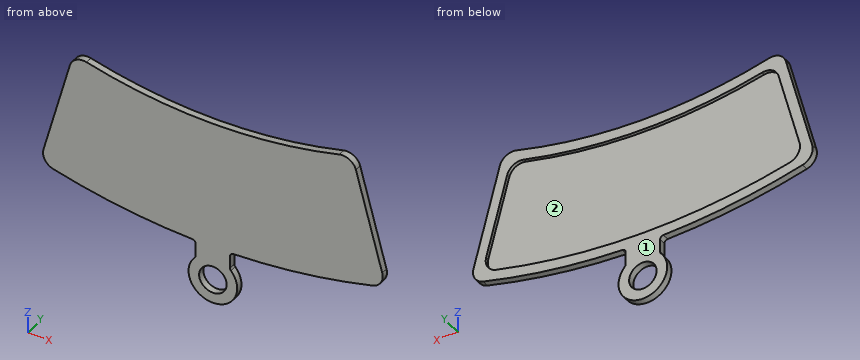
from build123d import *

# Parameters (mm, degrees)
BOSS_EXTRUDE1_DEPTH   = 1
CUT_EXTRUDE2_DEPTH    = 0.5
FILLET2_R             = 2
FILLET3_R             = 0.5
F_4_0MM_DOWEL_HOLE1_D = 4


with BuildPart() as part:
    # Sketch1 → Boss-Extrude1 (new body)
    with BuildSketch(Plane(origin=(0, 0, 0), x_dir=(1, 0, 0), z_dir=(0, 1, 0))):
        with BuildLine():
            Line((-25.127648951, 87.982107603), (-20.261027783, 69.819630142))
            ThreePointArc((-20.261027783, 69.819630142), (0, 72.7), (20.261027783, 69.819630142))
            Line((20.261027783, 69.819630142), (25.127648951, 87.982107603))
            ThreePointArc((25.127648951, 87.982107603), (13.92309714, 90.434492126), (2.499766704, 91.465846995))
            Line((2.499766704, 91.465846995), (2.499766704, 94))
            ThreePointArc((2.499766704, 94), (0.000164965, 100.03536894), (-2.5, 94.000233296))
            Line((-2.5, 94.000233296), (-2.5, 91.465840618))
            ThreePointArc((-2.5, 91.465840618), (-13.923212473, 90.434474369), (-25.127648951, 87.982107603))
        make_face()
    extrude(amount=BOSS_EXTRUDE1_DEPTH)

    # Sketch2 → Cut-Extrude2 (cut)
    with BuildSketch(Plane(origin=(0, 1, 0), x_dir=(1, 0, 0), z_dir=(0, 1, 0))):
        with BuildLine():
            Line((19.204373147, 71.671696311), (23.293714059, 86.933324366))
            ThreePointArc((23.293714059, 86.933324366), (0, 90), (-23.293714059, 86.933324366))
            Line((-23.293714059, 86.933324366), (-19.204373147, 71.671696311))
            ThreePointArc((-19.204373147, 71.671696311), (0, 74.2), (19.204373147, 71.671696311))
        make_face()
    extrude(amount=-CUT_EXTRUDE2_DEPTH, mode=Mode.SUBTRACT)

    # Fillet2
    fillet2_edges = [part.edges().sort_by_distance(p)[0] for p in [
        (25.127648951, 0.5, -87.982107603),
        (20.261027783, 0.5, -69.819630142),
        (-20.261027783, 0.5, -69.819630142),
        (-25.127648951, 0.5, -87.982107603),
        (19.204373147, 0.75, -71.671696311),
        (-19.204373147, 0.75, -71.671696311),
        (-23.293714059, 0.75, -86.933324366),
        (23.293714059, 0.75, -86.933324366),
    ]]
    fillet(fillet2_edges, radius=FILLET2_R)

    # Fillet3
    fillet3_edges = [part.edges().sort_by_distance(p)[0] for p in [
        (-2.5, 0.5, -91.465840618),
        (-2.5, 0.5, -94.000233296),
        (2.499766704, 0.5, -94),
        (2.499766704, 0.5, -91.465846995),
    ]]
    fillet(fillet3_edges, radius=FILLET3_R)

    # Ø4.0mm Dowel Hole1 (through all)
    with Locations(Plane(origin=(0, 1, 0), x_dir=(1, 0, 0), z_dir=(0, 1, 0))):
        with Locations((0, 96.5)):
            Hole(F_4_0MM_DOWEL_HOLE1_D / 2)


solid = part.part
Work out the finished part from the listing and answer in its coordinate system (mm). Face numbers are marked on the shaded views. Coordinates: 2 decimals unless noted, no trailing zeros. Loops run counter-clockwise (first coordinate to the right, second up) from the corner with the lowest first, then second, coordinate; pieces in that order, holes last. Notation, with made-up numbers: M 15,-8 L 29,-8 A25 ccw 29,21 Z; hole C 27.5,18.25 d2. An arc over 180 degrees is marked long. Answer in a Markdown table with one row per item. Add a question column.
1. Find section D-D, the plane x = 15.5. Write down the section's boundary in (y, z).
2. Find section B-B, the plane x = 0. Write down the section's boundary in (y, z), then the cut area to 3 significant figures.
3. Consider L1, parallel to X at y = 0.8, z = -96.5; L2, parallel to Y at x = -16, z = -80; L3, parallel to X at y = 0.45, z = -86.5. Determine where each line is inside the solid, lowest interval first.
4. Find section A-A, the plane z = -96.5. Write down the section's boundary in (x, y).
5. The mould has two halves that part along Z. Classify the marked faces 1 and 2: pulls with the +Z half, pulls with the -Z half, needs draft (parallel to the pull), parting line crosses it, or undercut.
6. Flat-ended cylindrical pins translate along their axes: P1, Ø14.5, axis at x = -3.5, z = -82, coming from the +Y side; P2, Ø4.5, axis at x = 0, z = -96.5, coming from the +Y side. Find the tip coordinate at first contact, or state that the pin passes through.
7. Find section C-C, the plane y = 0.7. Write down the section's boundary in (x, z), then the cut area to 3 significant figures.
Reported:
| question | item | result |
|---|---|---|
| 1 | outline | M 0,-90.18 L 1,-90.18 L 1,-88.66 L 0.5,-88.66 L 0.5,-72.56 L 1,-72.56 L 1,-71.03 L 0,-71.03 Z |
| 2 | outline | M 0,-100.04 L 1,-100.04 L 1,-98.5 L 0,-98.5 Z; M 0,-94.5 L 1,-94.5 L 1,-90 L 0.5,-90 L 0.5,-74.2 L 1,-74.2 L 1,-72.7 L 0,-72.7 Z |
| 2 | area | 15.4 mm^2 |
| 3 | L1 | x = -3.54 to -2, 2 to 3.54 |
| 3 | L2 | y = 0 to 0.5 |
| 3 | L3 | x = -24.68 to 24.68 |
| 4 | outline | M -3.54,0 L -2,0 L -2,1 L -3.54,1 Z; M 2,0 L 3.54,0 L 3.54,1 L 2,1 Z |
| 5 | face 1 | needs draft |
| 5 | face 2 | undercut |
| 6 | P1 | stops at y = 0.5 |
| 6 | P2 | stops at y = 1 |
| 7 | outline | M -24.61,-86.06 A2 ccw -23.19,-88.51 A91.5 ccw -2.98,-91.45 A0.5 cw -2.5,-91.95 L -2.5,-93.8 A0.5 cw -2.63,-94.14 A3.54 ccw long 2.63,-94.14 A0.5 cw 2.5,-93.8 L 2.5,-91.95 A0.5 cw 2.98,-91.45 A91.5 ccw 23.19,-88.51 A2 ccw 24.61,-86.06 L 20.78,-71.76 A2 ccw 18.35,-70.35 A72.7 cw -18.35,-70.35 A2 ccw -20.78,-71.76 Z; hole M -22.77,-84.98 A2 ccw -21.31,-87.44 A90 ccw 21.31,-87.44 A2 ccw 22.77,-84.98 L 19.72,-73.58 A2 ccw 17.32,-72.15 A74.2 cw -17.32,-72.15 A2 ccw -19.72,-73.58 Z; hole C 0,-96.5 d4 |
| 7 | area | 221 mm^2 |
